Geometry: final body of the model. Coordinates: model frame, mm. Face numbers are marked on the shaded views. A direction names the side the tool comes from. Give positions to 0.01 mm unless a question says otherwise; leave off trailing zeros. Write each loop counter-clockwise with the first axis right and the second up, starting at its lowest first coordinate (ties: lowest second). Pieces come first, ordered by that corner, then holes. Notation, with made-up numbers: (-31, -34) - (-4, -34) arc R15 ccw to (-4, -6) - close; hole circle Ø5 at (61.5, -9). An arc over 180 degrees is marked (long way). Use CSV: the item, a comma, the result in double quotes. Start each with the question number.
(1) Section D-D on y = 0. Output: boundary loops of the cut face in (x, z).
(2) Section C-C on z = 2. Output: boundary loops of the cut face in (x, y), and give its area (3 significant figures).
(3) Reachability of the marked faces 1, 2, 3 and 4 from +Z, -Z, +X, -X, +Y, -Y: full face, straight path, thin tool, end or side. Return the list, or none.
(4) Section A-A on x = 0. Output: boundary loops of the cut face in (y, z).
(5) First-contact query: pin 1 Ø0.8 at (y, z) = (0, -1) entering from +X; pin 2 Ø1.1 at (x, z) = (5, -2.5) entering from -Y; pin 3 Ø3 at (x, z) = (2, 2) entering from -Y. Flat tips, straight axial feed; report the tip coordinate or a pass-through.
(6) Draft query along Z for the marked faces 5, 6, 7 and 8. Return one class per face: released by +Z, released by -Z, zero draft, split by the parting line, or undercut.
(7) Section B-B on x = 1.5. Output: boundary loops of the cut face in (y, z), and give its area (3 significant figures).
(8) Line query: probe 1 along Y at (x, z) = (0, 2.25); probe 2 along X at (y, z) = (-0.3, -2.25); probe 3 along Z at (x, y) = (0.5, 1.8). Output: solid intervals per line, ascending. Write a range as [from, to].
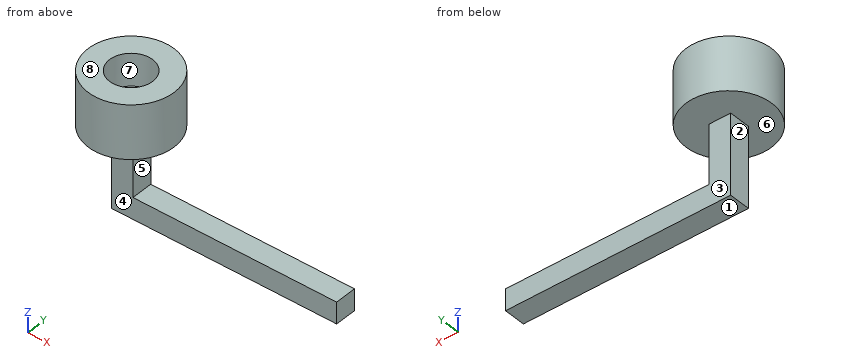
from build123d import *

# Parameters (mm, degrees)
SKETCH1_R           = 2
BOSS_EXTRUDE1_DEPTH = 2.5
SHELL1_T            = -1
SKETCH2_W           = 1
SKETCH2_H           = 1
BOSS_EXTRUDE2_DEPTH = 3.75
SKETCH3_W           = 1
SKETCH3_H           = 1
BOSS_EXTRUDE3_DEPTH = 9.5


with BuildPart() as part:
    # Sketch1 → Boss-Extrude1 (new body)
    with BuildSketch(Plane.XY):
        Circle(SKETCH1_R)
    extrude(amount=BOSS_EXTRUDE1_DEPTH)

    # Shell1
    shell1_openings = [part.faces().sort_by_distance(p)[0] for p in [
        (0, 0, 2.5),
    ]]
    offset(amount=SHELL1_T, openings=shell1_openings, kind=Kind.INTERSECTION)

    # Sketch2 → Boss-Extrude2 (add)
    with BuildSketch(Plane(origin=(0, 0, 0), x_dir=(-1, 0, 0), z_dir=(0, 0, -1))):
        Rectangle(SKETCH2_W, SKETCH2_H)
    extrude(amount=BOSS_EXTRUDE2_DEPTH)

    # Sketch3 → Boss-Extrude3 (add)
    with BuildSketch(Plane(origin=(0.5, 0, 0), x_dir=(0, 0, -1), z_dir=(1, 0, 0))):
        with Locations((3.25, 0)):
            Rectangle(SKETCH3_W, SKETCH3_H)
    extrude(amount=BOSS_EXTRUDE3_DEPTH)


solid = part.part
Check values:
1,outline,"(-2, 0) - (-0.5, 0) - (-0.5, -3.75) - (10, -3.75) - (10, -2.75) - (0.5, -2.75) - (0.5, 0) - (2, 0) - (2, 2.5) - (1, 2.5) - (1, 1) - (-1, 1) - (-1, 2.5) - (-2, 2.5) - close"
2,outline,"circle Ø4 at (0, 0); hole circle Ø2 at (0, 0)"
2,area,"9.42 mm²"
3,face 1,"-Z, +X, -X, +Y, -Y"
3,face 2,"-Z, -X, +Y, -Y"
3,face 3,"-Z, +X, -X, +Y"
3,face 4,"-Z, +X, -X, -Y"
4,outline,"(-2, 0) - (-0.5, 0) - (-0.5, -3.75) - (0.5, -3.75) - (0.5, 0) - (2, 0) - (2, 2.5) - (1, 2.5) - (1, 1) - (-1, 1) - (-1, 2.5) - (-2, 2.5) - close"
5,pin 1,"stops at x = 0.5"
5,pin 2,"stops at y = -0.5"
5,pin 3,"stops at y = -1.94"
6,face 5,"undercut"
6,face 6,"undercut"
6,face 7,"zero draft"
6,face 8,"released by +Z"
7,outline,"(-1.32, 0) - (1.32, 0) - (1.32, 2.5) - (-1.32, 2.5) - close; (-0.5, -3.75) - (0.5, -3.75) - (0.5, -2.75) - (-0.5, -2.75) - close"
7,area,"7.61 mm²"
8,probe 1,"y = [-2, -1], [1, 2]"
8,probe 2,"x = [-0.5, 0.5]"
8,probe 3,"z = [0, 2.5]"
